```python
from build123d import *

# Parameters (mm, degrees)
EXTRUDE_1_DEPTH     = 80
FILLET_1_R          = 10
CUT_EXTRUDE_1_DEPTH = 4
SKETCH_3_W          = 16
SKETCH_3_H          = 3
CUT_EXTRUDE_2_DEPTH = 4
CUT_EXTRUDE_3_REACH = 90.843
SKETCH_5_W          = 8
SKETCH_5_H          = 70
CUT_EXTRUDE_4_DEPTH = 1
FILLET_2_R          = 2


with BuildPart() as part:
    # Эскиз1 → Бобышка-Вытянуть1 (new body)
    with BuildSketch(Plane(origin=(0, 0, 0), x_dir=(1, 0, 0), z_dir=(0, 1, 0))):
        Polygon((0, 0), (-38, 0), (-38, 2), (-35.113248654, 7), (-2.886751346, 7), (0, 2), align=None)
    extrude(amount=EXTRUDE_1_DEPTH)

    # Скругление1
    fillet_1_edges = [part.edges().sort_by_distance(p)[0] for p in [
        (0, 0, -1),
        (-38, 0, -1),
        (-38, 80, -1),
        (0, 80, -1),
    ]]
    fillet(fillet_1_edges, radius=FILLET_1_R)

    # Эскиз2 → Вырез-Вытянуть1 (cut)
    with BuildSketch(Plane.XY):
        with BuildLine():
            Line((-28, 3), (-10, 3))
            ThreePointArc((-10, 3), (-5.050252532, 5.050252532), (-3, 10))
            Line((-3, 10), (-3, 70))
            ThreePointArc((-3, 70), (-5.050252532, 74.949747468), (-10, 77))
            Line((-10, 77), (-28, 77))
            ThreePointArc((-28, 77), (-32.949747468, 74.949747468), (-35, 70))
            Line((-35, 70), (-35, 10))
            ThreePointArc((-35, 10), (-32.949747468, 5.050252532), (-28, 3))
        make_face()
    extrude(amount=-CUT_EXTRUDE_1_DEPTH, mode=Mode.SUBTRACT)

    # Эскиз3 → Вырез-Вытянуть2 (cut)
    with BuildSketch(Plane.XY):
        with Locations((-19, 78.5)):
            Rectangle(SKETCH_3_W, SKETCH_3_H)
        with Locations((-19, 1.5)):
            Rectangle(SKETCH_3_W, SKETCH_3_H)
    extrude(amount=-CUT_EXTRUDE_2_DEPTH, mode=Mode.SUBTRACT)

    # Эскиз4 → Вырез-Вытянуть3 (cut, up to next)
    with BuildSketch(Plane(origin=(0, 0, -7), x_dir=(-1, 0, 0), z_dir=(0, 0, -1)), mode=Mode.PRIVATE) as cut_extrude_3_sk1:
        with BuildLine():
            Line((21.35, 70), (21.35, 10))
            ThreePointArc((21.35, 10), (19, 7.65), (16.65, 10))
            Line((16.65, 10), (16.65, 70))
            ThreePointArc((16.65, 70), (19, 72.35), (21.35, 70))
        make_face()
    cut_extrude_3_tool1 = extrude(cut_extrude_3_sk1.sketch, amount=-CUT_EXTRUDE_3_REACH, mode=Mode.PRIVATE) & part.part
    add(cut_extrude_3_tool1.solids().sort_by_distance((-19, 40, -7))[0], mode=Mode.SUBTRACT)

    # Эскиз5 → Вырез-Вытянуть4 (cut)
    with BuildSketch(Plane(origin=(0, 0, -7), x_dir=(-1, 0, 0), z_dir=(0, 0, -1))):
        with Locations((9.768375673, 40)):
            Rectangle(SKETCH_5_W, SKETCH_5_H)
        with Locations((28.231624327, 40)):
            Rectangle(SKETCH_5_W, SKETCH_5_H)
    extrude(amount=-CUT_EXTRUDE_4_DEPTH, mode=Mode.SUBTRACT)

    # Скругление2
    fillet_2_edges = [part.edges().sort_by_distance(p)[0] for p in [
        (-13.768375673, 75, -6.5),
        (-13.768375673, 5, -6.5),
        (-5.768375673, 5, -6.5),
        (-5.768375673, 75, -6.5),
        (-32.231624327, 75, -6.5),
        (-32.231624327, 5, -6.5),
        (-24.231624327, 5, -6.5),
        (-24.231624327, 75, -6.5),
    ]]
    fillet(fillet_2_edges, radius=FILLET_2_R)


solid = part.part
```
The model under review builds one solid part; all positions refer to its coordinate system, in mm. A direction names the side the tool comes from. Round coordinates to 2 decimals unless told otherwise and drop trailing zeros. Loops run counter-clockwise (first coordinate to the right, second up) from the corner with the lowest first, then second, coordinate; pieces in that order, holes last.
1) The part is to be moulded in two halves that separate along Y. For faces 1 (the face through (-4, 2, -3)), 2 (the face through (-19, 80, -5)), 3 (the face through (-33, 5.1, -2)), say which applies: pulls with the +Y half, pulls with the -Y half, needs draft (parallel to the pull), parting line crosses it, or undercut.
Values follow:
face 1: pulls with the -Y half
face 2: pulls with the +Y half
face 3: undercut
2) Consider section C-C on z = -3. State the section outline as (x, y) points, then the cut area to 3 significant figures.
Values follow:
outline: (-37.42, 6.65) arc R10 ccw to (-28, 0) - (-27, 0) - (-27, 3) - (-28, 3) arc R7 cw to (-35, 10) - (-35, 70) arc R7 cw to (-28, 77) - (-27, 77) - (-27, 80) - (-28, 80) arc R10 ccw to (-37.42, 73.35) - close; (-11, 0) - (-10, 0) arc R10 ccw to (-0.58, 6.65) - (-0.58, 73.35) arc R10 ccw to (-10, 80) - (-11, 80) - (-11, 77) - (-10, 77) arc R7 cw to (-3, 70) - (-3, 10) arc R7 cw to (-10, 3) - (-11, 3) - close
area: 458 mm2
3) Consider section D-D on x = -14.5. State the section outline as (y, z) points, then the cut area to 3 significant figures.
Values follow:
outline: (0, -7) - (80, -7) - (80, -4) - (0, -4) - close
area: 240 mm2
4) Tool access review of faces 4 (the face through (-19.05, 7.65, -5.52)), 5 (the face through (-27, 78, -2)), 6 (the face through (-5.1, 5, -2)), 7 (the face through (-31.63, 5.57, -6.49)): name each direction out of +Z, -Z, +X, -X, +Y, -Y from which nothing blocks a thin tool from reaching the whole face with its end or side.
Values follow:
face 4: +Z, -Z
face 5: +Z, +Y, -Y
face 6: +Z
face 7: -Z
5) Consider section A-A on x = -19. State the section outline as (y, z) points, then the cut area to 3 significant figures.
Values follow:
outline: (0, -7) - (7.65, -7) - (7.65, -4) - (0, -4) - close; (72.35, -7) - (80, -7) - (80, -4) - (72.35, -4) - close
area: 45.9 mm2
6) Consider section B-B on y = 44. State the section outline as (x, z) points, then the cut area to 3 significant figures.
Values follow:
outline: (-38, -2) - (-35.11, -7) - (-32.23, -7) - (-32.23, -6) - (-24.23, -6) - (-24.23, -7) - (-21.35, -7) - (-21.35, -4) - (-35, -4) - (-35, 0) - (-38, 0) - close; (-16.65, -7) - (-13.77, -7) - (-13.77, -6) - (-5.77, -6) - (-5.77, -7) - (-2.89, -7) - (0, -2) - (0, 0) - (-3, 0) - (-3, -4) - (-16.65, -4) - close
area: 93.5 mm2
7) Clearance check with flat-ended pins moving along their axes: P1, Ø2, axis at y = 25.5, z = -5, coming from the -X side; P2, Ø1.5, axis at y = 78.5, z = -3, coming from the -X side; P3, Ø3, axis at y = 17, z = -5.5, coming from the +X side. State where each tip first meets the part, or that it passes through.
Values follow:
P1: stops at x = -36.85
P2: stops at x = -34.32
P3: stops at x = -1.15
8) Wall thickness on line 1 along X through (y, z) = (67, -0.5); line 2 along Y through (x, z) = (-27, -6.5); line 3 along X through (y, z) = (14, -6.5): over which ranges is each line inside the solid? List them lowest first.
Values follow:
line 1: x = -38 to -35, -3 to 0
line 2: y = 0 to 5, 75 to 80
line 3: x = -35.4 to -32.23, -24.23 to -21.35, -16.65 to -13.77, -5.77 to -2.6
